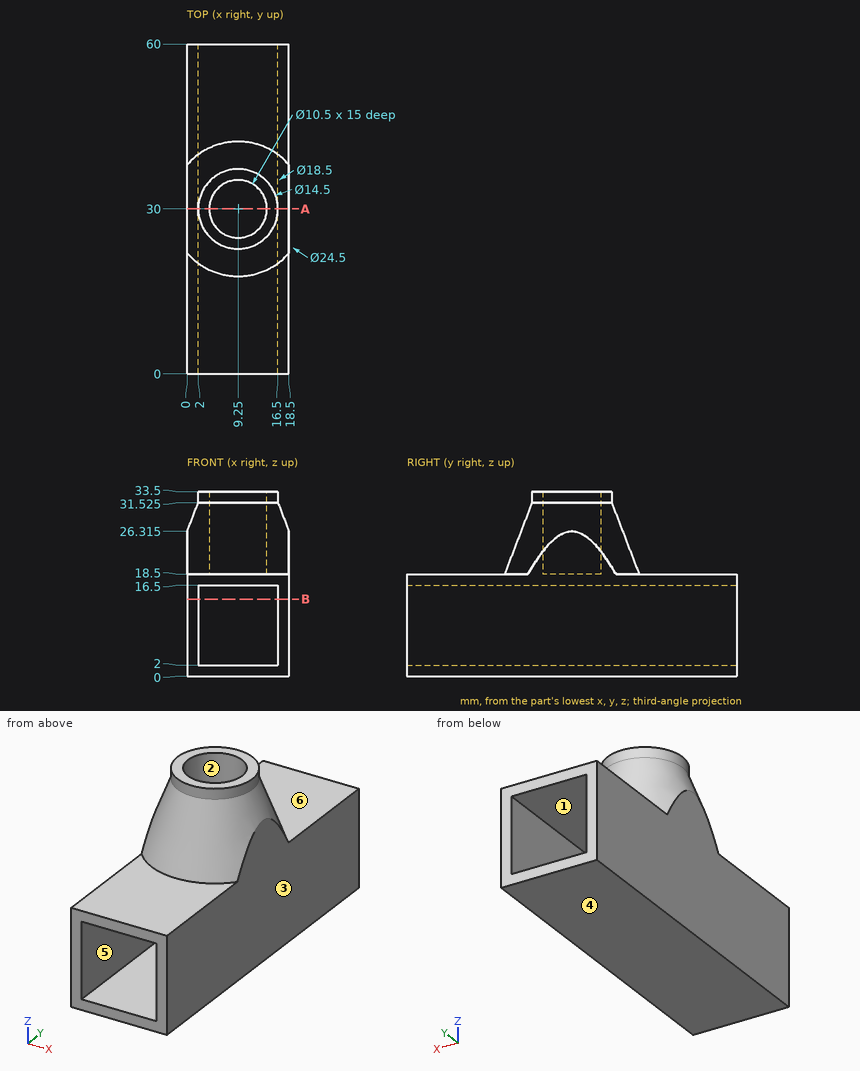
Input: dimensioned drawing with shaded views. Units: mm. Origin: part minimum x, y, z. A direction names the side the tool comes from. Coordinates: 2 decimals unless noted, no trailing zeros. Write each loop counter-clockwise with the first axis right and the second up, starting at its lowest first coordinate (ties: lowest second). Pieces come first, ordered by that corner, then holes. Notation, with made-up numbers: M 24,52.25 L 78,52.25 A9 cw 78,60.25 Z; hole C 1.5,-34.5 d8. An arc over 180 degrees is marked long. Answer as CSV lines item,"result". Start each with the question number.
Q1. Cut plane B-B on z = 14. Return the cut outline in (x, y).
Q2. Reachability of the marked faces 1, 2 and 3 from +Z, -Z, +X, -X, +Y, -Y: full face, straight path, thin tool, end or side. Return the list, or none.
Q3. Mould query, pull axis Z, two halves, no side actions, for the marked faces 4, 5 and 6. Classes: released by +Z, released by -Z, zero draft, split by the parting line, or undercut.
Q4. Cut plane A-A on y = 30. Return the cut outline in (x, z) (1 decimal).
Q5. Pin query (flat end, axial travel): P1, Ø6, axis at x = 14, z = 25.5, coming from the -Y side; P2, Ø5, axis at y = 28, z = 30, coming from the -X side; P3, Ø3, axis at y = 23, z = 29.5, coming from the +X side (1 decimal). Return the tip coordinate at first contact, or that it passes through.
Q6. Line query: line 1 (Z direction, x = 8, y = 27); line 2 (Z direction, x = 7.5, y = 24). Output: solid intervals per line, ascending. Write a range as from..to.
Findings below:
1,outline,"M 0,0 L 2,0 L 2,60 L 0,60 Z; M 16.5,0 L 18.5,0 L 18.5,60 L 16.5,60 Z"
2,face 1,"+Y, -Y"
2,face 2,"+Z"
2,face 3,"+Z, -Z, +X, +Y, -Y"
3,face 4,"released by -Z"
3,face 5,"undercut"
3,face 6,"released by +Z"
4,outline,"M 0,0 L 18.5,0 L 18.5,26.3 L 16.5,31.5 L 16.5,33.5 L 14.5,33.5 L 14.5,18.5 L 4,18.5 L 4,33.5 L 2,33.5 L 2,31.5 L 0,26.3 Z; hole M 2,2 L 16.5,2 L 16.5,16.5 L 2,16.5 Z"
5,P1,"stops at y = 19.94"
5,P2,"stops at x = 0.59"
5,P3,"stops at x = 15.3"
6,line 1,"z = 0..2, 16.5..18.5"
6,line 2,"z = 0..2, 16.5..33.5"
